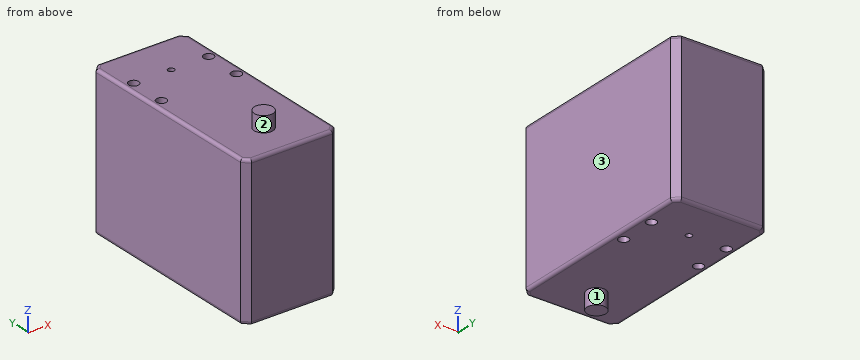
from build123d import *

# Parameters (mm, degrees)
SKETCH_1_W           = 30
SKETCH_1_H           = 65
EXTRUDE_1_DEPTH      = 48
SKETCH_2_R           = 1
CUT_EXTRUDE_1_DEPTH  = 48
EXTRUDE_2_DEPTH      = 5
EXTRUDE_2_DEPTH_BACK = 53
SKETCH_3_R           = 3
CHAMFER_1_SIZE       = 2
FILLET_1_R           = 1
FILLET_2_R           = 1
SKETCH_6_R           = 1.6
CUT_EXTRUDE_3_DEPTH  = 76


with BuildPart() as part:
    # Sketch 1 → Extrude 1 (new body)
    with BuildSketch(Plane.XY):
        with Locations((44.026916893, 39.150883092)):
            Rectangle(SKETCH_1_W, SKETCH_1_H)
    extrude(amount=EXTRUDE_1_DEPTH)

    # Sketch 2 → Cut-Extrude 1 (cut)
    with BuildSketch(Plane.XY):
        with Locations((56.026916893, 57.650883092)):
            Circle(SKETCH_2_R)
        with Locations((44.026916893, 57.650883092)):
            Circle(SKETCH_2_R)
        with Locations((56.023819064, 45.923533591)):
            Circle(SKETCH_2_R)
        with Locations((32.026916893, 57.650883092)):
            Circle(SKETCH_2_R)
        with Locations(Location((32.030014722, 45.923533591, 0), (0, 0, 180))):
            Circle(SKETCH_2_R)
    extrude(amount=CUT_EXTRUDE_1_DEPTH, mode=Mode.SUBTRACT)

    # Sketch 3 → Extrude 2 (add, two sides: drawn at the far end of the back side and taken through both)
    with BuildSketch(Plane(origin=(0, 0, 0), x_dir=(-1, 0, 0), z_dir=(0, 0, -1)).offset(-EXTRUDE_2_DEPTH_BACK)):
        with Locations((-44.026916893, 18.650883092)):
            Circle(SKETCH_3_R)
    extrude(amount=EXTRUDE_2_DEPTH + EXTRUDE_2_DEPTH_BACK)

    # Chamfer 1
    chamfer_1_edges = [part.edges().sort_by_distance(p)[0] for p in [
        (29.026916893, 71.650883092, 24),
        (59.026916893, 71.650883092, 24),
        (59.026916893, 6.650883092, 24),
        (29.026916893, 6.650883092, 24),
    ]]
    chamfer(chamfer_1_edges, length=CHAMFER_1_SIZE)

    # Fillet 1
    fillet_1_edges = [part.edges().sort_by_distance(p)[0] for p in [
        (44.026916893, 6.650883092, 48),
        (29.026916893, 39.150883092, 48),
        (59.026916893, 39.150883092, 48),
        (44.026916893, 71.650883092, 48),
        (30.026916893, 70.650883092, 48),
        (58.026916893, 70.650883092, 48),
        (58.026916893, 7.650883092, 48),
        (30.026916893, 7.650883092, 48),
    ]]
    fillet(fillet_1_edges, radius=FILLET_1_R)

    # Fillet 2
    fillet_2_edges = [part.edges().sort_by_distance(p)[0] for p in [
        (44.026916893, 6.650883092, 0),
        (29.026916893, 39.150883092, 0),
        (44.026916893, 71.650883092, 0),
        (59.026916893, 39.150883092, 0),
        (30.026916893, 70.650883092, 0),
        (58.026916893, 70.650883092, 0),
        (58.026916893, 7.650883092, 0),
        (30.026916893, 7.650883092, 0),
    ]]
    fillet(fillet_2_edges, radius=FILLET_2_R)

    # Sketch 6 → Cut-Extrude 3 (cut)
    with BuildSketch(Plane(origin=(0, 0, 0), x_dir=(-1, 0, 0), z_dir=(0, 0, -1))):
        with Locations((-55.99912174, 57.606952707)):
            Circle(SKETCH_6_R)
        with Locations((-32.054712046, 57.694813478)):
            Circle(SKETCH_6_R)
        with Locations((-55.99912174, 45.879603206)):
            Circle(SKETCH_6_R)
        with Locations((-32.054712046, 45.967463976)):
            Circle(SKETCH_6_R)
    extrude(amount=-CUT_EXTRUDE_3_DEPTH, mode=Mode.SUBTRACT)


solid = part.part
Model file for the job. Use its own axes, mm. Face numbers are marked on the shaded views. A direction names the side the tool comes from. Give positions to 0.01 mm unless a question says otherwise; leave off trailing zeros. Order: outer loops, then holes, each group sorted by start corner. A loop starts at its lowest first (then second) coordinate and runs counter-clockwise, first axis right, second up. Notation, with made-up numbers: M 31.25,76 L 37.25,76 A28 cw 37.25,108 Z; hole C -19.75,-19.5 d10. An arc over 180 degrees is marked long. Put each result on its own line as item: value. Start each with the question number.
(1) Band-saw the part on B-B on x = 55.25. Give the cut face in (y, z).
(2) Band-saw the part on A-A on y = 34. Give the cut face in (x, z), then the cut area to 3 significant figures.
(3) Pin check, flat tips, straight feed: pin 1 Ø1.9 at (x, y) = (56, 57.61) entering from -Z; pin 2 Ø2 at (x, y) = (33, 50) entering from +Z; pin 3 Ø3 at (x, y) = (48.5, 34.5) entering from -Z. Stop position of each tip, or through.
(4) Band-saw the part on D-D on x = 52. Give the cut face in (y, z).
(5) Tool access for the marked faces 1, 2 and 3: list every direction of +Z, -Z, +X, -X, +Y, -Y with a clear straight run to the whole face (end or side of a thin tool).
(6) Band-saw the part on C-C on z = 33. Give the cut face in (x, y).
(7) Drill centre lines: L1, parallel to Y at x = 56, z = 40.5; L2, parallel to Y at x = 44, z = 23; L3, parallel to Y at x = 54.75, z = 46. Where is each one in solid material? Low to high. Write a range as [from, to].
Results below:
1. outline: M 6.65,1 A1 ccw 7.65,0 L 44.47,0 L 44.47,48 L 7.65,48 A1 ccw 6.65,47 Z; M 47.29,0 L 56.19,0 L 56.19,48 L 47.29,48 Z; M 59.02,0 L 70.65,0 A1 ccw 71.65,1 L 71.65,47 A1 ccw 70.65,48 L 59.02,48 Z
2. outline: M 29.03,1 A1 ccw 30.03,0 L 58.03,0 A1 ccw 59.03,1 L 59.03,47 A1 ccw 58.03,48 L 30.03,48 A1 ccw 29.03,47 Z
2. area: 1,440 mm2
3. pin 1: passes through
3. pin 2: stops at z = 48
3. pin 3: stops at z = 0
4. outline: M 6.65,1 A1 ccw 7.65,0 L 70.65,0 A1 ccw 71.65,1 L 71.65,47 A1 ccw 70.65,48 L 7.65,48 A1 ccw 6.65,47 Z
5. face 1: -Z
5. face 2: +Z
5. face 3: +Z, -Z, +X, +Y, -Y
6. outline: M 29.03,8.65 L 31.03,6.65 L 57.03,6.65 L 59.03,8.65 L 59.03,69.65 L 57.03,71.65 L 31.03,71.65 L 29.03,69.65 Z; hole C 32.05,45.97 d3.2; hole C 32.05,57.69 d3.2; hole C 44.03,57.65 d2; hole C 56,45.88 d3.2; hole C 56,57.61 d3.2
7. L1: y = [6.65, 44.28], [47.48, 56.01], [59.21, 71.65]
7. L2: y = [6.65, 56.65], [58.65, 71.65]
7. L3: y = [6.65, 44.88], [46.88, 56.61], [58.61, 71.65]
